Source: CAD feature listing. Evaluate the final solid. Frame: model axes, mm. A direction names the side the tool comes from. Round coordinates to 2 decimals unless told otherwise and drop trailing zeros. Order: outer loops, then holes, each group sorted by start corner. A loop starts at its lowest first (then second) coordinate and runs counter-clockwise, first axis right, second up. Notation, with made-up numbers: (40.5, 31) - (81.5, 31) arc R30 ccw to (81.5, 70) - close; hole circle Ø3 at (71.5, -21). An arc over 180 degrees is marked (long way). Put each result on its own line as item: value. Start each with the question number.
1) Section B-B on x = -2. Output: boundary loops of the cut face in (y, z) (1 decimal).
2) Section A-A on x = 62. Output: boundary loops of the cut face in (y, z) (1 decimal), then the cut area to 3 significant figures.
3) Mould query, pull axis Y, two halves, no side actions, for faces 1 (the face through (-1, -62, -2)), 2 (the face through (1.04, 60.57, -3.4)), 3 (the face through (66.85, 59.65, 26.24)), 4 (the face through (58.54, 27.34, -2.35)). Classes: +Y half, -Y half, draft (parallel to the pull), parting line (faces both ways), or undercut.
4) Section C-C on z = 9. Output: boundary loops of the cut face in (x, y).
5) Access query for faces 5 (the face through (42.74, 59.65, 20.9)), 6 (the face through (-1, -2, -4.762)), 7 (the face through (-1, 57.238, 17)). Directions: +Z, -Z, +X, -X, +Y, -Y. A direction counts if a zero-diameter tool reaches every point of the face in a straight line with its end or side. Return the directions, or none.
6) Section D-D on y = -30. Output: boundary loops of the cut face in (x, z).
7) Line query: probe 1 along Y at (x, z) = (-62, -1); probe 2 along Z at (x, y) = (-18, -2); probe 3 along Y at (x, z) = (3, 16.5). Output: solid intervals per line, ascending. Write a range as [from, to].
8) Contact query for flat-ended pins moving along their axis: P1, Ø5, axis at x = 5.5, y = 59.5, coming from the +Z side; P2, Ø10, axis at x = 21.5, z = 8, coming from the -Y side; P3, Ø11.5, axis at x = 0, y = 30, coming from the +Z side; P4, Ø10, axis at x = -61.3, z = 26, coming from the +Y side. Output: stop coordinate, or through.
```python
from build123d import *

# Parameters (mm, degrees)
F0_R     = 4.365625
F0_W     = 148
F0_H     = 4.7625
F1_DEPTH = 4.7625
F2_DEPTH = 44
F3_R     = 4.7625
F4_R     = 5.55625
F5_DEPTH = 6.35


# Not quite as in the source:
# - a feature names something its author has since deleted; it is built from what else it names


with BuildPart() as f1:
    # F0 (on Top) → F1 (new body)
    with BuildSketch(Plane.XY):
        with BuildLine():
            Line((-31, -12.365625), (-31, -62))
            Line((-31, -62), (0, -62))
            Line((0, -62), (74, -62))
            Line((74, -62), (74, 57.2375))
            Line((74, 57.2375), (-74, 57.2375))
            Line((-74, 57.2375), (-74, -8))
            Line((-74, -8), (-62, -8))
            Line((-62, -8), (-35.365625, -8))
            ThreePointArc((-35.365625, -8), (-31, -3.634375), (-26.634375, -8))
            ThreePointArc((-26.634375, -8), (-27.9130369584, -11.0869630416), (-31, -12.365625))
        make_face()
        with BuildLine():
            ThreePointArc((4.365625, -49), (3.0869630416, -52.0869630416), (0, -53.365625))
            ThreePointArc((0, -53.365625), (-4.365625, -49), (0, -44.634375))
            ThreePointArc((0, -44.634375), (3.0869630416, -45.9130369584), (4.365625, -49))
        make_face(mode=Mode.SUBTRACT)
        with Locations((62, -46)):
            Circle(F0_R, mode=Mode.SUBTRACT)
        with Locations((31, -8)):
            Circle(F0_R, mode=Mode.SUBTRACT)
        with BuildLine():
            ThreePointArc((-57.634375, 30), (-58.9130369584, 26.9130369584), (-62, 25.634375))
            ThreePointArc((-62, 25.634375), (-65.0869630416, 33.0869630416), (-57.634375, 30))
        make_face(mode=Mode.SUBTRACT)
        with BuildLine():
            ThreePointArc((4.365625, 30), (3.0869630416, 26.9130369584), (0, 25.634375))
            ThreePointArc((0, 25.634375), (-3.0869630416, 33.0869630416), (4.365625, 30))
        make_face(mode=Mode.SUBTRACT)
        with Locations((62, 30)):
            Circle(F0_R, mode=Mode.SUBTRACT)
        with Locations((0, 59.61875)):
            Rectangle(F0_W, F0_H)
        with BuildLine():
            Line((-62, -50.365625), (-62, -62))
            Line((-62, -62), (-31, -62))
            Line((-31, -62), (-31, -12.365625))
            ThreePointArc((-31, -12.365625), (-34.0869630416, -11.0869630416), (-35.365625, -8))
            Line((-35.365625, -8), (-62, -8))
            Line((-62, -8), (-62, -41.634375))
            ThreePointArc((-62, -41.634375), (-58.9130369584, -42.9130369584), (-57.634375, -46))
            ThreePointArc((-57.634375, -46), (-58.9130369584, -49.0869630416), (-62, -50.365625))
        make_face()
        with BuildLine():
            Line((-74, -8), (-74, -46))
            Line((-74, -46), (-66.365625, -46))
            ThreePointArc((-66.365625, -46), (-65.0869630416, -42.9130369584), (-62, -41.634375))
            Line((-62, -41.634375), (-62, -8))
            Line((-62, -8), (-74, -8))
        make_face()
        with BuildLine():
            Line((-74, -46), (-74, -62))
            Line((-74, -62), (-62, -62))
            Line((-62, -62), (-62, -50.365625))
            ThreePointArc((-62, -50.365625), (-65.0869630416, -49.0869630416), (-66.365625, -46))
            Line((-66.365625, -46), (-74, -46))
        make_face()
    extrude(amount=-F1_DEPTH)

    # F0 (on Top) → F2 (join)
    with BuildSketch(Plane.XY):
        with Locations((0, 59.61875)):
            Rectangle(F0_W, F0_H)
    extrude(amount=F2_DEPTH)

    # F3
    f3_edges = [f1.edges().sort_by_distance(p)[0] for p in [
        (0, 62, -4.7625),
    ]]
    fillet(f3_edges, radius=F3_R)

    # F4 (on face) → F5 (cut)
    with BuildSketch(Plane(origin=(0, 62, 0), x_dir=(-1, 0, 0), z_dir=(0, 1, 0))):
        with BuildLine():
            ThreePointArc((-60, 44), (-50.1005050634, 39.8994949366), (-46, 30))
            Line((-46, 30), (-46, 28.8925))
            ThreePointArc((-46, 28.8925), (-42.652230509, 20.810269491), (-34.57, 17.4625))
            Line((-34.57, 17.4625), (0, 17.4625))
            Line((0, 17.4625), (34.57, 17.4625))
            ThreePointArc((34.57, 17.4625), (42.652230509, 20.810269491), (46, 28.8925))
            Line((46, 28.8925), (46, 30))
            ThreePointArc((46, 30), (50.1005050634, 39.8994949366), (60, 44))
            Line((60, 44), (59.7125, 44))
            Line((59.7125, 44), (-60, 44))
        make_face()
        with BuildLine():
            Line((74, 44), (60, 44))
            ThreePointArc((60, 44), (69.8994949366, 39.8994949366), (74, 30))
            Line((74, 30), (74, 44))
        make_face()
        with Locations((-61.3, 26)):
            Circle(F4_R)
        with Locations((61.3, 26)):
            Circle(F4_R)
        with BuildLine():
            ThreePointArc((-74, 30), (-69.8994949366, 39.8994949366), (-60, 44))
            Line((-60, 44), (-74, 44))
            Line((-74, 44), (-74, 30))
        make_face()
    extrude(amount=-F5_DEPTH, mode=Mode.SUBTRACT)


solid = f1.part
```
Answer sheet:
1. outline: (-62, -4.8) - (-52.9, -4.8) - (-52.9, 0) - (-62, 0) - close; (-45.1, -4.8) - (26.1, -4.8) - (26.1, 0) - (-45.1, 0) - close; (33.9, -4.8) - (57.2, -4.8) arc R4.8 ccw to (62, 0) - (62, 17.5) - (57.2, 17.5) - (57.2, 0) - (33.9, 0) - close
2. outline: (-62, -4.8) - (-50.4, -4.8) - (-50.4, 0) - (-62, 0) - close; (-41.6, -4.8) - (25.6, -4.8) - (25.6, 0) - (-41.6, 0) - close; (34.4, -4.8) - (57.2, -4.8) arc R4.8 ccw to (62, 0) - (62, 20.5) - (57.2, 20.5) - (57.2, 0) - (34.4, 0) - close; (57.2, 31.5) - (62, 31.5) - (62, 43.9) - (57.2, 43.9) - close
2. area: 659 mm^2
3. face 1: -Y half
3. face 2: +Y half
3. face 3: draft
3. face 4: undercut
4. outline: (-74, 57.24) - (74, 57.24) - (74, 62) - (-74, 62) - close
5. face 5: +Z, +Y, -Y
5. face 6: -Z, +X, -X, +Y, -Y
5. face 7: +Z, +X, -X, -Y
6. outline: (-74, -4.76) - (74, -4.76) - (74, 0) - (-74, 0) - close
7. probe 1: [-62, -50.37], [-41.63, 25.63], [34.37, 61.89]
7. probe 2: [-4.76, 0]
7. probe 3: [57.24, 62]
8. P1: z = 17.46
8. P2: y = 57.24
8. P3: z = 0
8. P4: through
